from build123d import *

# Parameters (mm, degrees)
F1_DEPTH = 63.5
F0_W     = 25.2179650775
F0_H     = 19.05
F2_DEPTH = 25.4
F3_DEPTH = 7.9375
F5_R     = 6.35


# Not quite as in the source:
# - a feature names something its author has since deleted; it is built from what else it names


with BuildPart() as f1:
    # F0 (on Front) → F1 (new body, symmetric)
    with BuildSketch(Plane.XZ):
        Polygon((22.225, 9.525), (-41.275, 9.525), (-41.275, -9.525), (41.275, -9.525), (41.275, 9.525), align=None)
    extrude(amount=F1_DEPTH, both=True)

    # F0 (on Front) → F2 (join, symmetric)
    with BuildSketch(Plane.XZ):
        with BuildLine():
            Line((22.225, 27.0002), (22.225, 9.525))
            Line((22.225, 9.525), (41.275, 9.525))
            Line((41.275, 9.525), (41.275, 27.0002))
            ThreePointArc((41.275, 27.0002), (45.9246798487, 38.2255201513), (57.15, 42.8752))
            Line((57.15, 42.8752), (60.325, 42.8752))
            Line((60.325, 42.8752), (60.325, 61.9252))
            Line((60.325, 61.9252), (57.15, 61.9252))
            add(Edge.make_bspline(
                [(56.0083765395, 61.9065364001), (56.3896340439, 61.9145223536), (56.7701888152, 61.920748032), (57.15, 61.9252)],
                knots=[110.545873998, 110.545873998, 110.545873998, 110.545873998, 111.5045361635, 111.5045361635, 111.5045361635, 111.5045361635], degree=3))
            ThreePointArc((56.0083765395, 61.9065364001), (32.0539163976, 51.2889260436), (22.225, 27.0002))
        make_face()
        with Locations((72.9339825387, 52.4002)):
            Rectangle(F0_W, F0_H)
    extrude(amount=F2_DEPTH, both=True)

    # F0 (on Front) → F3 (join, symmetric)
    with BuildSketch(Plane.XZ):
        with BuildLine():
            add(Edge.make_bspline(
                [(-41.275, 9.525), (-41.2634975333, 36.6583816825), (12.04456367, 60.9856549384), (56.0083765395, 61.9065364001)],
                knots=[0, 0, 0, 0, 110.545873998, 110.545873998, 110.545873998, 110.545873998], degree=3))
            Line((-41.275, 9.525), (22.225, 9.525))
            Line((22.225, 9.525), (22.225, 27.0002))
            ThreePointArc((22.225, 27.0002), (32.0539163976, 51.2889260436), (56.0083765395, 61.9065364001))
        make_face()
    extrude(amount=F3_DEPTH, both=True)

    # F0 (on Front) → F4 (revolve)
    with BuildSketch(Plane.XZ):
        Polygon((85.5429650775, 66.675), (85.5429650775, 61.9252), (85.5429650775, 42.8752), (85.5429650775, 38.1), (111.125, 38.1), (111.125, 66.675), align=None)
    revolve(axis=Axis((85.5429650775, 0, 52.3875), (0, 0, -1)))

    # F5
    f5_edges = [f1.edges().sort_by_distance(p)[0] for p in [
        (41.275, -63.5, 0),
        (-41.275, -63.5, 0),
        (41.275, 63.5, 0),
        (-41.275, 63.5, 0),
    ]]
    fillet(f5_edges, radius=F5_R)


solid = f1.part
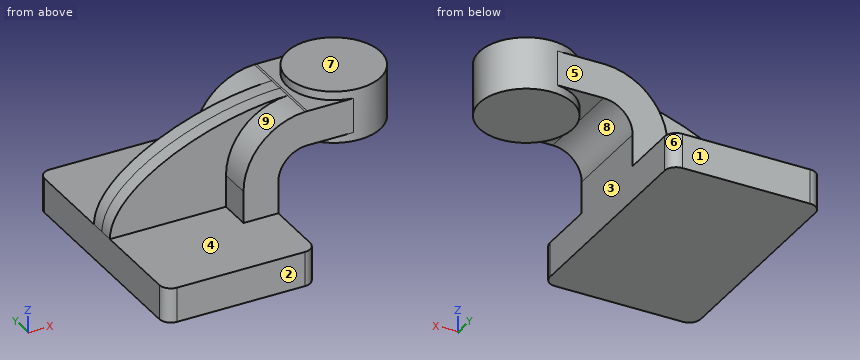
Design review of the part built by this model. Coordinates are the model's own, in mm. Face numbers are marked on the shaded views. A direction names the side the tool comes from. Coordinates: 2 decimals unless noted, no trailing zeros. Order: outer loops, then holes, each group sorted by start corner. A loop starts at its lowest first (then second) coordinate and runs counter-clockwise, first axis right, second up.
Item 1: For the marked faces 1, 2, 3, 4 and 5, list the 3-axis set-ups (+Z, -Z, +X, -X, +Y, -Y) from which the entire face can be reached by the end or side of a thin tool; tool diameter is ignored.
Item 2: For pin 1 Ø16.5 at (x, y) = (-7.5, 29.5) entering from +Z (3 decimals); pin 2 Ø10 at (y, z) = (-41.5, 4.5) entering from +X (3 decimals); pin 3 Ø14 at (y, z) = (17.5, 18) entering from -X (3 decimals), all flat-tipped, find the tip position at first contact; note any pin that passes through.
Item 3: Take a section at A-A, the plane y = 51. Write out the cut boundary in (x, z) (3 decimals).
Item 4: For line 1 (Y direction, x = 44, z = 56); line 2 (Z direction, x = -12, y = -31) (3 decimals); line 3 (X direction, y = 24, z = 18.5) (3 decimals), list the stretches that pass through material, from the lowest coordinate up.
Item 5: The part is to be moulded in two halves that separate along X. For the marked faces 6, 7, 8 and 9, say which applies: pulls with the +X half, pulls with the -X half, needs draft (parallel to the pull), parting line crosses it, or undercut.
The answers:
1. face 1: +Z, -Z, +X, -X, +Y
1. face 2: +Z, -Z, +X, -X, -Y
1. face 3: -Z, +X, +Y, -Y
1. face 4: +Z, -X, -Y
1. face 5: +Z, -X, +Y
2. pin 1: stops at z = 9.525
2. pin 2: stops at x = 41.275
2. pin 3: stops at x = 22.225
3. outline: (-41.275, -9.525) - (41.275, -9.525) - (41.275, 9.525) - (-41.275, 9.525) - close
4. line 1: y = -25.4 to 25.4
4. line 2: z = -9.525 to 9.525
4. line 3: x = 22.225 to 41.275
5. face 6: pulls with the +X half
5. face 7: needs draft
5. face 8: undercut
5. face 9: pulls with the -X half
